Geometry check sheet. Reference: the model listing, model coordinates, mm. Face numbers are marked on the shaded views. A direction names the side the tool comes from. Coordinates: 2 decimals unless noted, no trailing zeros. Loops run counter-clockwise (first coordinate to the right, second up) from the corner with the lowest first, then second, coordinate; pieces in that order, holes last. Notation, with made-up numbers: (18, -2) - (28, -2) arc R11 cw to (28, 7) - close; hole circle Ø8 at (32, -39.5). An arc over 180 degrees is marked (long way). One line per item, written item: value.
from build123d import *

# Parameters (mm, degrees)
F0_W      = 138.3
F0_H      = 67.1
F0_W_2    = 131.2
F0_H_2    = 60
F1_DEPTH  = 14.2
F2_R      = 5
F3_W      = 132.005408
F3_H      = 60.05396
F3_R      = 13.2201
F4_DEPTH  = 0.2
F5_R      = 2.967269
F5_R_2    = 2.980013
F6_DEPTH  = 1.5
F7_W      = 13.59712
F7_H      = 5.098922
F8_DEPTH  = 1.5
F9_R      = 3.740527
F10_DEPTH = 24
F11_W     = 15.491804
F11_H     = 7.459016
F12_DEPTH = 25


with BuildPart() as f1:
    # F0 (on Top) → F1 (new body)
    with BuildSketch(Plane.XY):
        Rectangle(F0_W, F0_H)
        Rectangle(F0_W_2, F0_H_2, mode=Mode.SUBTRACT)
    extrude(amount=F1_DEPTH)

    # F2
    f2_edges = [f1.edges().sort_by_distance(p)[0] for p in [
        (69.15, 33.55, 7.1),
        (69.15, -33.55, 7.1),
        (-69.15, -33.55, 7.1),
        (-69.15, 33.55, 7.1),
    ]]
    fillet(f2_edges, radius=F2_R)

    # F3 (on Top) → F4 (join)
    with BuildSketch(Plane.XY):
        Rectangle(F3_W, F3_H)
        with Locations((-19.262591, 0)):
            Circle(F3_R, mode=Mode.SUBTRACT)
        with BuildLine():
            ThreePointArc((-62.320147, 25.777878), (-58.637593, 29.460432), (-54.955039, 25.777878))
            Line((-54.955039, 25.777878), (-54.955039, 8.781476))
            ThreePointArc((-54.955039, 8.781476), (-58.637593, 5.098922), (-62.320147, 8.781476))
            Line((-62.320147, 8.781476), (-62.320147, 25.777878))
        make_face(mode=Mode.SUBTRACT)
    extrude(amount=-F4_DEPTH)

    # F5 (on face) → F6 (join)
    with BuildSketch(Plane.XZ.offset(33.55)):
        with Locations((-53.682171, 6.325473)):
            Circle(F5_R)
        with Locations((-44.906233, 5.765563)):
            Circle(F5_R_2)
    extrude(amount=F6_DEPTH)

    # F7 (on face) → F8 (join)
    with BuildSketch(Plane(origin=(-69.15, 0, 0), x_dir=(0, -1, 0), z_dir=(-1, 0, 0))):
        with Locations((17.279675, 7.648382)):
            Rectangle(F7_W, F7_H)
        with BuildLine():
            Line((24.078235, 10.197843), (24.078235, 5.098921))
            ThreePointArc((24.078235, 5.098921), (26.627696, 7.648382), (24.078235, 10.197843))
        make_face()
        with BuildLine():
            ThreePointArc((10.481115, 10.197843), (7.931654, 7.648382), (10.481115, 5.098921))
            Line((10.481115, 5.098921), (10.481115, 10.197843))
        make_face()
    extrude(amount=F8_DEPTH)

    # F9 (on face) → F10 (cut)
    with BuildSketch(Plane(origin=(-69.15, 0, 0), x_dir=(0, -1, 0), z_dir=(-1, 0, 0))):
        with Locations((-16.065575, 7.315574)):
            Circle(F9_R)
    extrude(amount=-F10_DEPTH, mode=Mode.SUBTRACT)

    # F11 (on face) → F12 (cut)
    with BuildSketch(Plane.YZ.offset(69.15)):
        with Locations((0, 8.17623)):
            Rectangle(F11_W, F11_H)
    extrude(amount=-F12_DEPTH, mode=Mode.SUBTRACT)


solid = f1.part
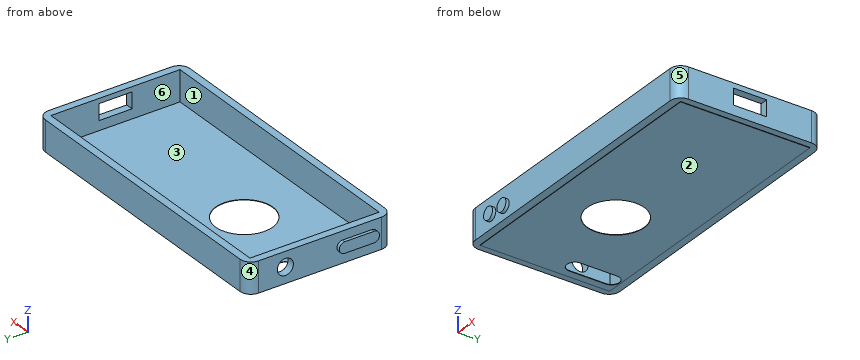
(1) Cross-section at A-A on y = 0. Record the cut outline in (x, z), and give its area (3 significant figures).
Reply:
outline: (-69.15, 0) - (-66, 0) - (-66, -0.2) - (-32.48, -0.2) - (-32.48, 0) - (-65.6, 0) - (-65.6, 14.2) - (-69.15, 14.2) - close; (-6.04, -0.2) - (66, -0.2) - (66, 0) - (69.15, 0) - (69.15, 4.45) - (65.6, 4.45) - (65.6, 0) - (-6.04, 0) - close; (65.6, 11.91) - (69.15, 11.91) - (69.15, 14.2) - (65.6, 14.2) - close
area: 95.5 mm2
(2) Cross-section at B-B on x = -13. Record the cut outline in (y, z), and give its area (3 significant figures).
Reply:
outline: (-33.55, 0) - (-30.03, 0) - (-30.03, -0.2) - (-11.64, -0.2) - (-11.64, 0) - (-30, 0) - (-30, 14.2) - (-33.55, 14.2) - close; (11.64, -0.2) - (30.03, -0.2) - (30.03, 0) - (33.55, 0) - (33.55, 14.2) - (30, 14.2) - (30, 0) - (11.64, 0) - close
area: 108 mm2
(3) Material ranges on probe 1 along X at (y, z) = (-7, 4.25); probe 2 along Y at (x, z) = (23, 2.25); probe 3 along X at (y, z) = (-20, 8), recorded low to high. Write a range as from..to.
Reply:
probe 1: -69.15..-65.6, 65.6..69.15
probe 2: -33.55..-30, 30..33.55
probe 3: -70.65..-65.6, 65.6..69.15
(4) Cross-section at C-C on y = 22.5. Record the cut outline in (x, z), and give its area (3 significant figures).
Reply:
outline: (-69.15, 0) - (-66, 0) - (-66, -0.2) - (-62.32, -0.2) - (-62.32, 0) - (-65.6, 0) - (-65.6, 14.2) - (-69.15, 14.2) - close; (-54.96, -0.2) - (66, -0.2) - (66, 0) - (69.15, 0) - (69.15, 14.2) - (65.6, 14.2) - (65.6, 0) - (-54.96, 0) - close
area: 126 mm2
(5) Go/stop test with flat-tipped pins: pin 1 Ø8 at (x, y) = (-38, -23.5) entering from +Z; pin 2 Ø7 at (x, z) = (26, 7.5) entering from -Y; pin 3 Ø4 at (x, z) = (67.5, 9) entering from +Y. Record where each tip stops, or that it passes through.
Reply:
pin 1: z = 0
pin 2: y = -33.55
pin 3: y = 33.36
(6) Release check for a two-part mould opening along X. For the marked faces 1, 2, 3 and 4 record: pulls with the +X half, pulls with the -X half, needs draft (parallel to the pull), parting line crosses it, or undercut.
Reply:
face 1: undercut
face 2: needs draft
face 3: undercut
face 4: pulls with the -X half
(7) Cross-section at D-D on x = 29.5. Record the cut outline in (y, z), and give its area (3 significant figures).
Reply:
outline: (-33.55, 0) - (-30.03, 0) - (-30.03, -0.2) - (30.03, -0.2) - (30.03, 0) - (33.55, 0) - (33.55, 14.2) - (30, 14.2) - (30, 0) - (-30, 0) - (-30, 14.2) - (-33.55, 14.2) - close
area: 113 mm2
(8) Access from +Z, -Z, +X, -X, +Y, -Y to the whole of each face (thin tool, end or side, straight path). Record for the marked faces 5 and 6.
Reply:
face 5: +Z, -Z, +X, -Y
face 6: +Z
